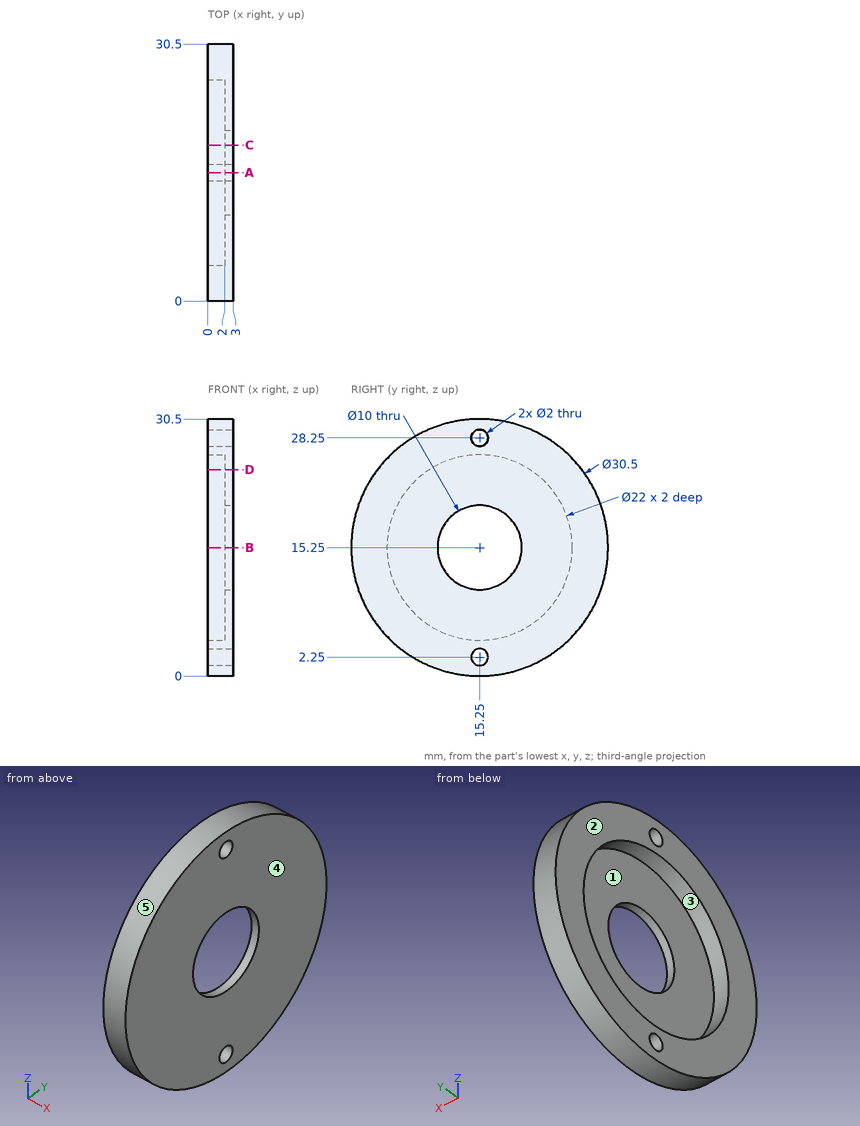
For this review, use the dimensioned drawing (mm, ordinates from the lowest corner) and the shaded views. A direction names the side the tool comes from. Round coordinates to 2 decimals unless told otherwise and drop trailing zeros. Order: outer loops, then holes, each group sorted by start corner. A loop starts at its lowest first (then second) coordinate and runs counter-clockwise, first axis right, second up. Notation, with made-up numbers: (35.5, -32.5) -> (75.5, -32.5) arc R34 ccw to (75.5, 3.5) -> close; hole circle Ø5 at (-6, 42). An arc over 180 degrees is marked (long way). Use CSV: the item, a comma, the result in double quotes. Start each with the question number.
(1) Consider section C-C on y = 18.5. Write out the cut boundary in (x, z).
(2) Insertion check: pin 1 (1.5 mm diameter, centred on x = 0.5, z = 18.5, fed in from +Y); pin 2 (4 mm diameter, centred on y = 22.5, z = 10.5, fed in from -X); pin 3 (1 mm diameter, centred on x = 1, y = 4, fed in from +Z). Each pin has a flat end and moves straight along its axis. Give the tip position at first contact, or say it passes through.
(3) Mouldability with a two-part tool opening along Y and no side actions: class the marked faces 3, 4 and 5 as pulls with the +Y half, pulls with the -Y half, needs draft (parallel to the pull), parting line crosses it, or undercut.
(4) Consider section D-D on z = 24.5. Write out the cut boundary in (x, y), and give its area (3 significant figures).
(5) Wall thickness on probe 1 along Z at (x, y) = (0.5, 15.25); probe 2 along Z at (x, y) = (2.1, 15.25); probe 3 along Y at (x, z) = (1.4, 15): over which ranges is each line inside the solid? List them lowest first. Write a range as from..to.
(6) Consider section B-B on z = 15.25. Write out the cut boundary in (x, y), and give its area (3 significant figures).
(7) Consider section A-A on y = 15.25. Write out the cut boundary in (x, z).
(8) Tool access review of the marked faces 1 and 2: name each direction out of +Z, -Z, +X, -X, +Y, -Y from which nothing blocks a thin tool from reaching the whole face with its end or side.
Responses:
1,outline,"(0, 0.35) -> (3, 0.35) -> (3, 11.45) -> (2, 11.45) -> (2, 4.74) -> (0, 4.74) -> close; (0, 25.76) -> (2, 25.76) -> (2, 19.05) -> (3, 19.05) -> (3, 30.15) -> (0, 30.15) -> close"
2,pin 1,"y = 30.29"
2,pin 2,"x = 2"
2,pin 3,"z = 26.07"
3,face 3,"undercut"
3,face 4,"needs draft"
3,face 5,"parting line crosses it"
4,outline,"(0, 3.13) -> (3, 3.13) -> (3, 27.37) -> (0, 27.37) -> (0, 21.2) -> (2, 21.2) -> (2, 9.3) -> (0, 9.3) -> close"
4,area,"48.9 mm²"
5,probe 1,"0..1.25, 3.25..4.25, 26.25..27.25, 29.25..30.5"
5,probe 2,"0..1.25, 3.25..10.25, 20.25..27.25, 29.25..30.5"
5,probe 3,"0..4.25, 26.25..30.5"
6,outline,"(0, 0) -> (3, 0) -> (3, 10.25) -> (2, 10.25) -> (2, 4.25) -> (0, 4.25) -> close; (0, 26.25) -> (2, 26.25) -> (2, 20.25) -> (3, 20.25) -> (3, 30.5) -> (0, 30.5) -> close"
6,area,"37.5 mm²"
7,outline,"(0, 0) -> (3, 0) -> (3, 1.25) -> (0, 1.25) -> close; (0, 3.25) -> (3, 3.25) -> (3, 10.25) -> (2, 10.25) -> (2, 4.25) -> (0, 4.25) -> close; (0, 26.25) -> (2, 26.25) -> (2, 20.25) -> (3, 20.25) -> (3, 27.25) -> (0, 27.25) -> close; (0, 29.25) -> (3, 29.25) -> (3, 30.5) -> (0, 30.5) -> close"
8,face 1,"-X"
8,face 2,"+Z, -Z, -X, +Y, -Y"
